Autodesk Inventor part; units mm, degrees
ref_plane "YZ Plane" through (0, 0, 0) normal (1, 0, 0) x (0, 1, 0)
ref_plane "XZ Plane" through (0, 0, 0) normal (0, 1, 0) x (-1, 0, 0)
ref_plane "XY Plane" through (0, 0, 0) normal (0, 0, 1) x (1, 0, 0)
sketch "Sketch1" plane through (0, 0, 0) normal (0, 1, 0) x (-1, 0, 0)
  point P0 (0, 0)
sketch "Sketch2" plane through (0, 0, 0) normal (0, 1, 0) x (-1, 0, 0)
  circle A0 centre (0, 0) radius 10 construction
  arc A1 (5.0714, -10.8757) -> (5.0714, 10.8757) centre (0, 0) ccw
  line L0 (5.0714, 10.8757) -> (5.0714, -10.8757) construction
  line L1 (5.0714, 10.8757) -> (26.8228, 10.8757) construction
  line L2 (5.0714, -10.8757) -> (65.0714, -10.8757)
  line L3 (5.0714, -10.8757) -> (65.0714, -10.8757) construction
  line L4 (65.0714, -10.8757) -> (100.0714, -71.4975)
  line L5 (100.0714, -71.4975) -> (104.4015, -68.9975)
  line L6 (5.0714, 10.8757) -> (58.2868, 10.8757)
  line L7 (58.2868, 10.8757) -> (104.4015, -68.9975)
  dimension "d0" = 20
  dimension "d1" = 90
  dimension "d2" = 2
  dimension "d3" = 130
  dimension "d4" = 60
  dimension "d5" = 0
  dimension "d6" = 70
  dimension "d7" = 120
  dimension "d8" = 5
extrude "Extrusion1" add sketch "Sketch2" along normal blind 10
sketch "Sketch3" plane through (0, 10, 0) normal (0, 1, 0) x (1, 0, 0)
  line L0 (-58.2868, -10.8757) -> (-104.4015, 68.9975)
  line L1 (-58.2868, -10.8757) -> (-44.9829, -33.9186)
  arc A0 (-5.0714, 10.8757) -> (-5.0714, -10.8757) centre (0, 0) ccw
  line L2 (-44.9829, -33.9186) -> (-5.0714, -10.8757)
  line L3 (-58.2868, -10.8757) -> (-5.0714, -10.8757)
  line L4 (-58.2868, -10.8757) -> (-5.0714, -10.8757)
extrude "Extrusion2" add sketch "Sketch3" against normal blind 10
sketch "Sketch4" plane through (0, 0, 0) normal (0, -1, 0) x (1, 0, 0)
  circle A0 centre (-46.3227, 11.5981) radius 1.25
  circle A1 centre (-29.0022, 1.5981) radius 1.25
  line L0 (-29.0022, 1.5981) -> (-46.3227, 11.5981) construction
  line L1 (-44.9829, 33.9186) -> (-104.4015, -68.9975) construction
  line L2 (-5.0714, 10.8757) -> (-44.9829, 33.9186) construction
  point P0 (0, 0)
  dimension "d13" = 2.5
  dimension "d14" = 2.5
  dimension "d15" = 20
  dimension "d16" = 10
  dimension "d17" = 20
extrude "Extrusion3" cut sketch "Sketch4" along normal through all both and the other way through all
properties part number "flipper-hug-left"
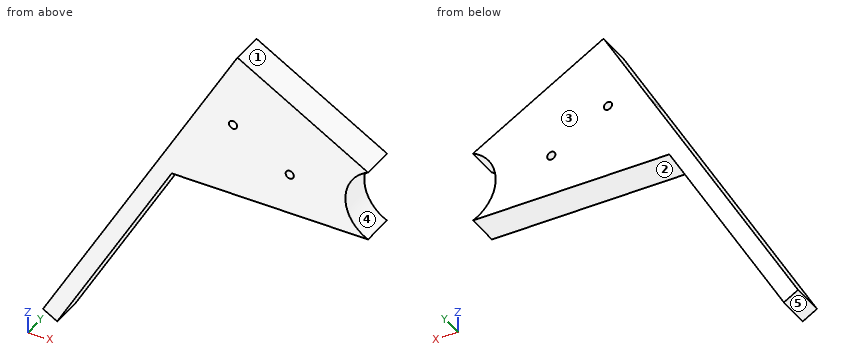
Geometry check sheet. Reference: the model listing, model coordinates, mm. Face numbers are marked on the shaded views. A direction names the side the tool comes from. Round coordinates to 2 decimals unless told otherwise and drop trailing zeros. Loops run counter-clockwise (first coordinate to the right, second up) from the corner with the lowest first, then second, coordinate; pieces in that order, holes last. Notation, with made-up numbers: (38, -38) -> (65, -38) arc R9 cw to (65, -22) -> close; hole circle Ø5 at (22.5, 27.5). An arc over 180 degrees is marked (long way). Answer as a JSON object with one key per item and string values. Group by question number.
Item 1: Thickness scan on line 1 along X through (y, z) = (5, -17.5); line 2 along X through (y, z) = (9.5, -55); line 3 along Z through (x, y) = (-71, 4). Record the ranges inside material, lowest first.
Item 2: Cross-section at A-A, the plane y = 5. Record the cut outline in (x, z), plus the area to 3 significant figures.
Item 3: Release check for a two-part mould opening along Z. For the marked faces 3, 4 and 5 record: pulls with the +Z half, pulls with the -Z half, needs draft (parallel to the pull), parting line crosses it, or undercut.
Item 4: Set-up check for the marked faces 1 and 2: record each of +Z, -Z, +X, -X, +Y, -Y from which the full face is reachable in a straight line by a thin tool's end or side.
Item 5: Cross-section at B-B, the plane z = -37.5. Record the cut outline in (x, y).
Item 6: Cross-section at C-C, the plane x = -88. Record the cut outline in (y, z), plus the area to 3 significant figures.
Item 7: Depth check by flat-ended pin: pin 1 Ø3 at (y, z) = (5.5, -42.5) entering from +X; pin 2 Ø10 at (x, z) = (-84.5, -56.5) entering from -Y; pin 3 Ø5 at (y, z) = (2, -32.5) entering from +X; pin 4 Ø2 at (y, z) = (1, 14.5) entering from +X. Enter the tip coordinate at first touch or a pass-through.
Determined:
{
 "1": {"line 1": "x = -74.67 to -68.9", "line 2": "x = -96.32 to -90.55", "line 3": "z = -21.14 to -11.14"},
 "2": {"outline": "(-104.4, -69) -> (-100.07, -71.5) -> (-65.07, -10.88) -> (-5.07, -10.88) arc R12 cw to (-5.07, 10.88) -> (-44.98, 33.92) -> (-58.29, 10.88) -> close; hole circle Ø2.5 at (-46.32, 11.6); hole circle Ø2.5 at (-29, 1.6)", "area": "2,130 mm²"},
 "3": {"face 3": "needs draft", "face 4": "undercut", "face 5": "pulls with the -Z half"},
 "4": {"face 1": "+Z, +X, +Y, -Y", "face 2": "-Z, +X, +Y, -Y"},
 "5": {"outline": "(-86.22, 0) -> (-80.44, 0) -> (-80.44, 10) -> (-86.22, 10) -> close"},
 "6": {"outline": "(0, -50.59) -> (10, -50.59) -> (10, -40.59) -> (0, -40.59) -> close", "area": "100 mm²"},
 "7": {"pin 1": "stops at x = -82.46", "pin 2": "passes through", "pin 3": "stops at x = -76.11", "pin 4": "stops at x = -9.62"}
}
